Answer from the drawing. Dimensions are ordinates in mm from the lowest x, y and z of the part. Coordinates: 2 decimals unless noted, no trailing zeros. Write each loop counter-clockwise with the first axis right and the second up, starting at its lowest first coordinate (ties: lowest second). Pieces come first, ordered by that corner, then holes.
(1) Straight lines are drawn through the part: line 1 (Y direction, x = 10, z = 9.25); line 2 (X direction, y = 7.5, z = 12.5); line 3 (Y direction, x = 5.5, z = 7.75). For each, find the intervals that lie inside material, in ascending order.
(2) Given P1, Ø3, axis at y = 3.5, z = 7.5, coming from the -X side; P2, Ø2, axis at y = 15, z = 18, coming from the -X side; P3, Ø8, axis at x = 10, y = 10, coming from the -Z side; P4, Ø1.5, axis at x = 18, z = 10, coming from the +Y side, each flat-ended and moving along its own axis, determine where each tip first touches the part or whether it passes through.
(3) For a pull along X with two mould halves and no side action, classify the marked faces 1, 2 and 3 as +X half, -X half, draft (parallel to the pull), parting line (faces both ways), or undercut.
(4) The part is cut by section C-C on z = 17.25. Determine the outline of the cut face in (x, y), plus the area to 3 significant figures.
(5) The part is cut by section A-A on y = 10. Determine the outline of the cut face in (x, z).
(6) The part is cut by section D-D on z = 2.5. Determine the outline of the cut face in (x, y).
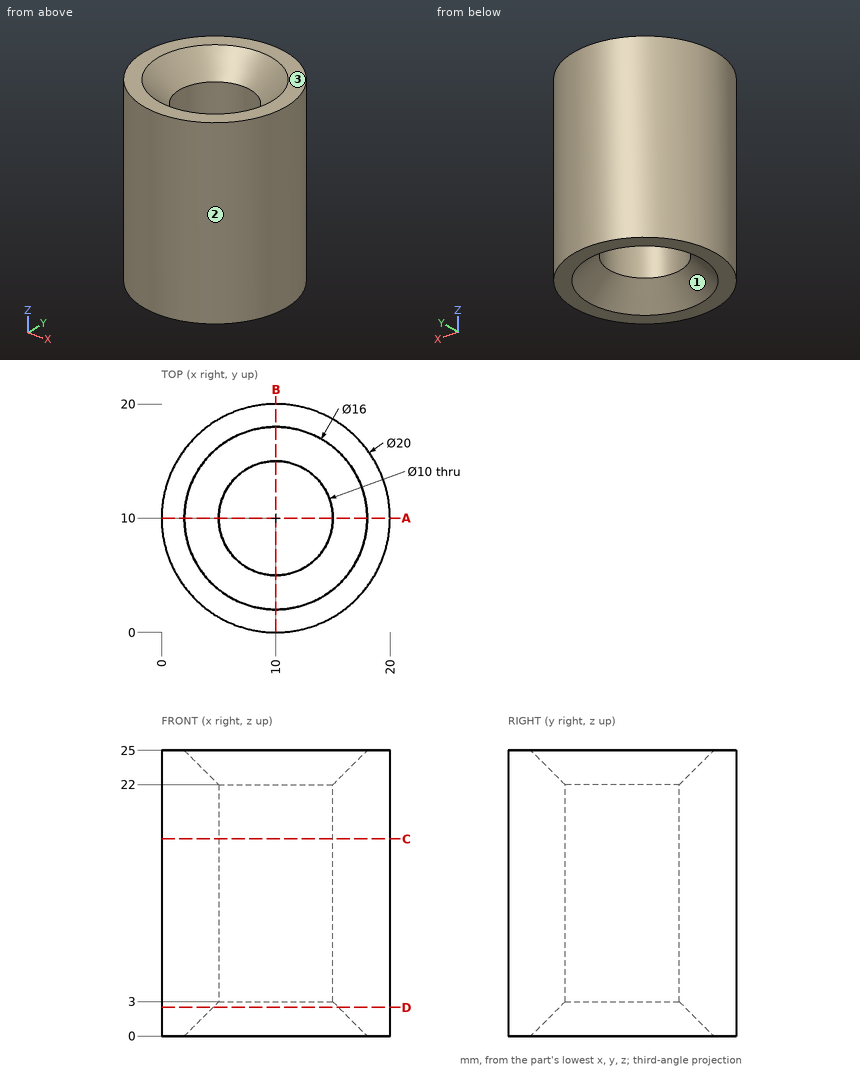
Model answer:
1. line 1: y = 0 to 5, 15 to 20
1. line 2: x = 0.32 to 5.67, 14.33 to 19.68
1. line 3: y = 1.07 to 7.82, 12.18 to 18.93
2. P1: stops at x = 1.34
2. P2: stops at x = 0.83
2. P3: passes through
2. P4: stops at y = 16.89
3. face 1: undercut
3. face 2: parting line
3. face 3: draft
4. outline: circle Ø20 at (10, 10); hole circle Ø10 at (10, 10)
4. area: 236 mm2
5. outline: (0, 0) - (2, 0) - (5, 3) - (5, 22) - (2, 25) - (0, 25) - close; (15, 3) - (18, 0) - (20, 0) - (20, 25) - (18, 25) - (15, 22) - close
6. outline: circle Ø20 at (10, 10); hole circle Ø11 at (10, 10)
